from build123d import *

# Parameters (mm, degrees)
F0_W     = 36
F0_H     = 10
F1_DEPTH = 2
F2_DEPTH = 4
F4_D     = 6
F4_DEPTH = 2


with BuildPart() as f1:
    # F0 (on Top) → F1 (new body)
    with BuildSketch(Plane.XY):
        Rectangle(F0_W, F0_H)
        Polygon((20, 7), (-20, 7), (-20, 5), (-18, 5), (18, 5), (20, 5), align=None)
        Polygon((-18, -5), (-20, -5), (-20, -7), (20, -7), (20, -5), (18, -5), align=None)
    extrude(amount=F1_DEPTH)

    # F0 (on Top) → F2 (join)
    with BuildSketch(Plane.XY):
        Polygon((20, 7), (-20, 7), (-20, 5), (-18, 5), (18, 5), (20, 5), align=None)
        Polygon((-18, -5), (-20, -5), (-20, -7), (20, -7), (20, -5), (18, -5), align=None)
    extrude(amount=F2_DEPTH)

    # F4
    with Locations(Plane(origin=(0, 0, 0), x_dir=(1, 0, 0), z_dir=(0, 0, -1))):
        with Locations((0, 0)):
            Hole(F4_D / 2, depth=F4_DEPTH)


solid = f1.part
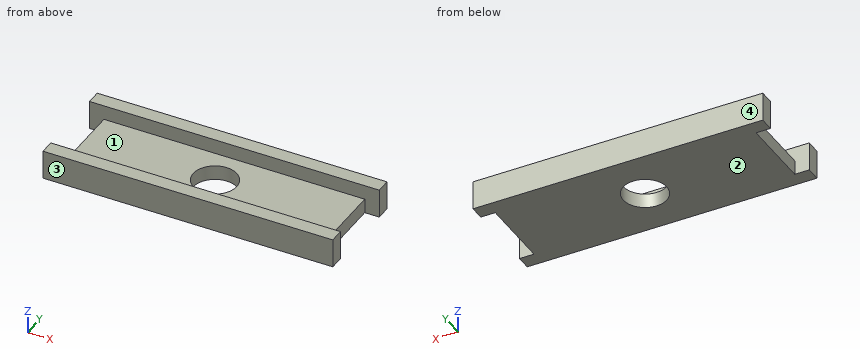
Geometry: final body of the model. Coordinates: model frame, mm. Face numbers are marked on the shaded views. Round coordinates to 2 decimals unless told otherwise and drop trailing zeros. Write each loop counter-clockwise with the first axis right and the second up, starting at its lowest first coordinate (ties: lowest second). Pieces come first, ordered by that corner, then holes. Notation, with made-up numbers: M -35.5,-29 L 10.5,-29 A15 cw 10.5,-7 Z; hole C -26,-11 d5. An arc over 180 degrees is marked long. Write item = value, one per line.
Item 1: Section query C-C on z = 2.9. Return loops of the section in (x, y), then the cut area to 3 significant figures.
Findings:
outline = M -20,-7 L 20,-7 L 20,-5 L -20,-5 Z; M -20,5 L 20,5 L 20,7 L -20,7 Z
area = 160 mm^2
Item 2: Pin query (flat end, axial travel): P1, Ø2, axis at y = -2, z = 0.5, coming from the -X side; P2, Ø2, axis at y = 1.5, z = 1.5, coming from the +X side. Return the tip coordinate at first contact, or that it passes through.
Findings:
P1 = -18
P2 = 18
Item 3: Section query D-D on x = 4. Return loops of the section in (y, z).
Findings:
outline = M -7,0 L 7,0 L 7,4 L 5,4 L 5,2 L -5,2 L -5,4 L -7,4 Z
Item 4: Section query B-B on x = 0. Return loops of the section in (y, z), then the cut area to 3 significant figures.
Findings:
outline = M -7,0 L -3,0 L -3,2 L -5,2 L -5,4 L -7,4 Z; M 3,0 L 7,0 L 7,4 L 5,4 L 5,2 L 3,2 Z
area = 24.0 mm^2
Item 5: Pull-direction query (Y, two-part tool) for the marked faces 1, 2, 3 and 4; classes: pulls with the +Y half, pulls with the -Y half, needs draft (parallel to the pull), parting line crosses it, or undercut.
Findings:
face_1 = undercut
face_2 = needs draft
face_3 = pulls with the -Y half
face_4 = pulls with the +Y half
Item 6: Section query A-A on y = 0. Return loops of the section in (x, z).
Findings:
outline = M -18,0 L -3,0 L -3,2 L -18,2 Z; M 3,0 L 18,0 L 18,2 L 3,2 Z
Item 7: Material intervals for line 1 along Y through (x, z) = (0, 0.9); line 2 along Y through (x, z) = (-0.5, 3.7); line 3 along X through (y, z) = (-4, 0.6), sorted ascending. Write a range as [from, to].
Findings:
line_1 = [-7, -3], [3, 7]
line_2 = [-7, -5], [5, 7]
line_3 = [-18, 18]
